Job drawing, mm, ordinate dimensions from the low corner. One solid piece. Round coordinates to 2 decimals unless told otherwise and drop trailing zeros. Loops run counter-clockwise (first coordinate to the right, second up) from the corner with the lowest first, then second, coordinate; pieces in that order, holes last.
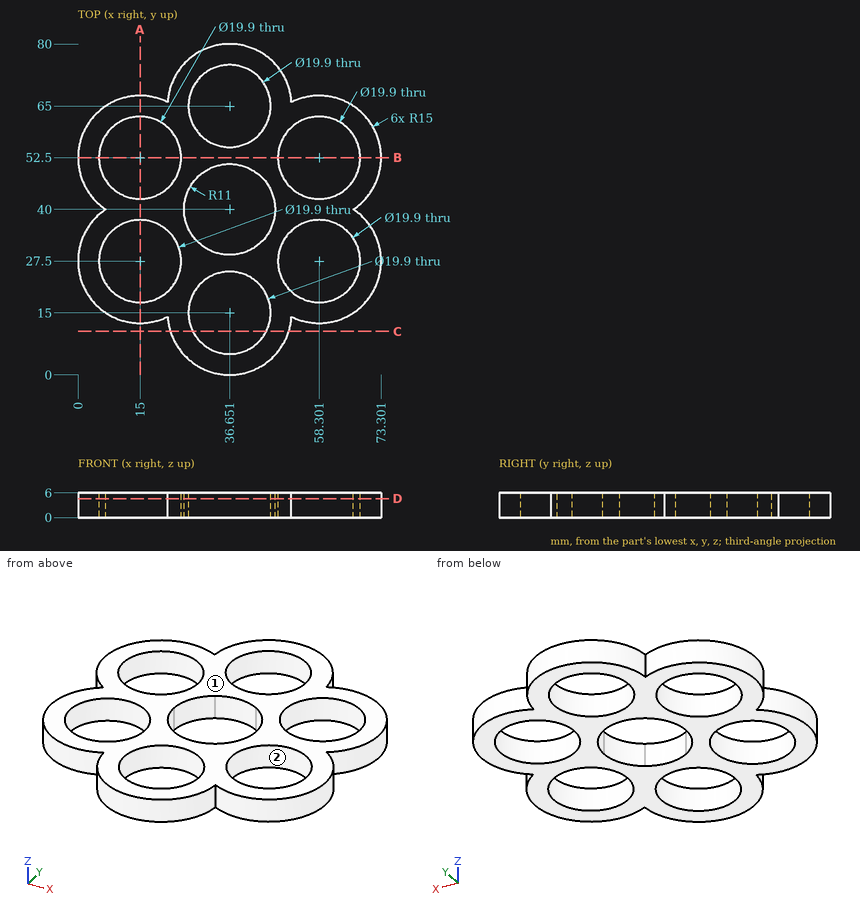
1) Drop flat-ended pins along their axis: pin 1 Ø1 at (y, z) = (57.5, 4) entering from -X; pin 2 Ø1.5 at (y, z) = (39, 2) entering from -X; pin 3 Ø1 at (y, z) = (56, 1.5) entering from -X. Give the stop position or say it passes through.
Values:
pin 1: stops at x = 0.69
pin 2: stops at x = 4.54
pin 3: stops at x = 0.3
2) Mould opens along X. For the marked faces 1 and 2 say: released by +X, released by -X, zero draft, split by the parting line, or undercut.
Values:
face 1: zero draft
face 2: undercut
3) Slice it at D-D, the plane z = 4.6. Give the cut face in (x, y), then the cut area to 3 significant figures.
Values:
outline: (6.71, 40) arc R15 ccw to (21.68, 14.07) arc R15 ccw to (51.62, 14.07) arc R15 ccw to (66.59, 40) arc R15 ccw to (51.62, 65.93) arc R15 ccw to (21.68, 65.93) arc R15 ccw to start; hole circle Ø19.9 at (15, 27.5); hole circle Ø19.9 at (15, 52.5); hole (25.65, 40) arc R11 ccw to (31.15, 30.47) arc R11 ccw to (42.15, 30.47) arc R11 ccw to (47.65, 40) arc R11 ccw to (42.15, 49.53) arc R11 ccw to (31.15, 49.53) arc R11 ccw to start; hole circle Ø19.9 at (36.65, 15); hole circle Ø19.9 at (36.65, 65); hole circle Ø19.9 at (58.3, 27.5); hole circle Ø19.9 at (58.3, 52.5)
area: 2,040 mm2
4) Slice it at B-B, the plane y = 52.5. Give the cut face in (x, z).
Values:
outline: (0, 0) - (5.05, 0) - (5.05, 6) - (0, 6) - close; (24.95, 0) - (48.35, 0) - (48.35, 6) - (24.95, 6) - close; (68.25, 0) - (73.3, 0) - (73.3, 6) - (68.25, 6) - close
5) Slice it at C-C, the plane y = 10.5. Give the cut face in (x, z) (1 decimal).
Values:
outline: (22.3, 0) - (27.8, 0) - (27.8, 6) - (22.3, 6) - close; (45.5, 0) - (51, 0) - (51, 6) - (45.5, 6) - close
6) Slice it at A-A, the plane x = 15. Give the cut face in (y, z), then the cut area to 3 significant figures.
Values:
outline: (12.5, 0) - (17.55, 0) - (17.55, 6) - (12.5, 6) - close; (37.45, 0) - (42.55, 0) - (42.55, 6) - (37.45, 6) - close; (62.45, 0) - (67.5, 0) - (67.5, 6) - (62.45, 6) - close
area: 91.2 mm2
7) Wall check: line 1 along Y through (x, z) = (15, 3.8); line 2 along Y through (x, z) = (19, 2.95); line 3 along Y through (x, z) = (31.5, 4.55). Give the ranges that are in metal, low to high.
Values:
line 1: y = 12.5 to 17.55, 37.45 to 42.55, 62.45 to 67.5
line 2: y = 13.04 to 18.39, 36.61 to 43.39, 61.61 to 66.96
line 3: y = 0.91 to 6.49, 23.51 to 30.28, 49.72 to 56.49, 73.51 to 79.09
